The listing builds one solid part. Answer for the finished solid, in the listing's coordinates (mm). A direction names the side the tool comes from. Give positions to 0.01 mm unless a question says otherwise; leave off trailing zeros. Order: outer loops, then holes, each group sorted by start corner. A loop starts at its lowest first (then second) coordinate and runs counter-clockwise, first axis right, second up. Notation, with made-up numbers: (-10, 59) - (35, 59) arc R26 cw to (35, 86) - close; hole circle Ø11 at (29.5, 7.25). An arc over 180 degrees is marked (long way). Answer in a Markdown table with one row per item.
from build123d import *

# Parameters (mm, degrees)
SKETCH_2_R          = 4.5
SKETCH_2_R_2        = 2.5
CUT_EXTRUDE_1_DEPTH = 0.2
CHAMFER_1_SIZE      = 0.2
CUT_EXTRUDE_START   = -0.2
SKETCH_3_R          = 4.5
SKETCH_3_R_2        = 2.5
CUT_EXTRUDE_2_DEPTH = 0.2
CHAMFER_2_SIZE      = 0.2


with BuildPart() as part:
    # 草图1 → 旋转1 (revolve)
    with BuildSketch(Plane.XY, mode=Mode.PRIVATE) as revolve_1_sk:
        Polygon((-2, 1.5), (-2, 6), (-1.4, 6), (0, 4.6), (1.4, 6), (2, 6), (2, 1.5), align=None)
    revolve(revolve_1_sk.sketch.rotate(Axis((-2, 0, 0), (1, 0, 0)), 90), axis=Axis((-2, 0, 0), (1, 0, 0)))

    # 草图2 → 切除-拉伸1 (cut)
    with BuildSketch(Plane(origin=(2, 0, 0), x_dir=(0, 0, -1), z_dir=(1, 0, 0))):
        Circle(SKETCH_2_R)
        Circle(SKETCH_2_R_2, mode=Mode.SUBTRACT)
    extrude(amount=-CUT_EXTRUDE_1_DEPTH, mode=Mode.SUBTRACT)

    # 倒角1
    chamfer_1_edges = [part.edges().sort_by_distance(p)[0] for p in [
        (2, 0, 4.5),
    ]]
    chamfer(chamfer_1_edges, length=CHAMFER_1_SIZE - 0.0001)  # a hair under: the kernel refuses the full size

    # 草图3 → 切除-拉伸2 (cut)
    with BuildSketch(Plane.ZY.offset(2).offset(CUT_EXTRUDE_START)):
        Circle(SKETCH_3_R)
        with Locations(Location((0, 0, 0), (0, 0, 180))):
            Circle(SKETCH_3_R_2, mode=Mode.SUBTRACT)
    extrude(amount=CUT_EXTRUDE_2_DEPTH, mode=Mode.SUBTRACT)

    # 倒角2
    chamfer_2_edges = [part.edges().sort_by_distance(p)[0] for p in [
        (-2, 0, -4.5),
    ]]
    chamfer(chamfer_2_edges, length=CHAMFER_2_SIZE - 0.0001)  # a hair under: the kernel refuses the full size


solid = part.part
Item 1: Each of these flat-tipped pins is pushed along its axis until it touches: P1, Ø5, axis at y = 0, z = 0, coming from the +X side; P2, Ø2, axis at x = 0, z = 3, coming from the -Y side. Where does it stop, or does it pass through?
Answer block:
| item | result |
|---|---|
| P1 | x = 2 |
| P2 | y = -4.87 |
Item 2: Consider line 1 (X direction, y = 2.5, z = -0.5); line 2 (X direction, y = 1, z = 5); line 3 (X direction, y = 0.25, z = -5.25). Determine where each line is inside the solid, lowest interval first.
Answer block:
| item | result |
|---|---|
| line 1 | -1.8 to 1.8 |
| line 2 | -2 to -0.5, 0.5 to 2 |
| line 3 | -2 to -0.66, 0.66 to 2 |
Item 3: Find section C-C on x = 0.75. Write down the section's boundary in (y, z).
Answer block:
| item | result |
|---|---|
| outline | circle Ø10.7 at (0, 0); hole circle Ø3 at (0, 0) |
Item 4: Which of the six approach directions +Z, -Z, +X, -X, +Y, -Y give full straight-line access (tool end or side, diameter ignored) to faces 1 (the face through (-1.696, -1.802, 5.723)), 2 (the face through (-1.8, -2, 2)), 3 (the face through (1.8, -2, -2))?
Answer block:
| item | result |
|---|---|
| face 1 | +X, -X |
| face 2 | -X |
| face 3 | +X |
